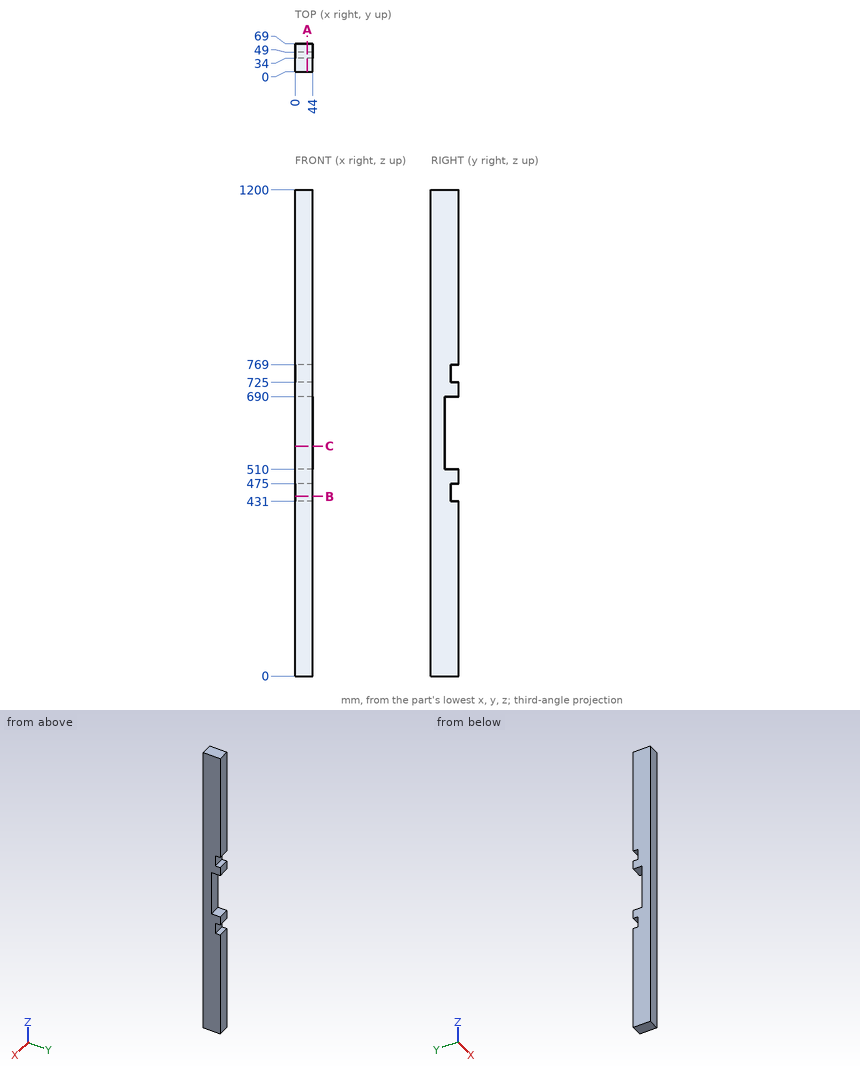
For this review, use the dimensioned drawing (mm, ordinates from the lowest corner) and the shaded views. Coordinates: 2 decimals unless noted, no trailing zeros. Write each loop counter-clockwise with the first axis right and the second up, starting at its lowest first coordinate (ties: lowest second). Pieces come first, ordered by that corner, then holes. Notation, with made-up numbers: (87, 4) -> (94, 4) arc R35 cw to (94, 43) -> close; hole circle Ø1 at (76.5, 12.25). An arc over 180 degrees is marked (long way). Write each question's results on one line, items separated by ' | '. Start each with the question number.
(1) Take a section at A-A on x = 30.5. Write out the cut boundary in (y, z), and give its area (3 significant figures).
(2) Take a section at B-B on z = 443.5. Write out the cut boundary in (x, y), and give its area (3 significant figures).
(3) For line 1 along Z through (x, y) = (34, 56); line 2 along Z through (x, y) = (2.5, 44.5); line 3 along Y through (x, z) = (11.5, 467), list the stretches that pass through material, from the lowest coordinate up. Write a range as from..to.
(4) Take a section at C-C on z = 567.5. Write out the cut boundary in (x, y), and give its area (3 significant figures).
(5) Clearance check with flat-ended pins moving along their axes: P1, Ø13, axis at x = 23.5, z = 558.5, coming from the +Y side; P2, Ø13, axis at x = 23, z = 444, coming from the +Y side. State where each tip first meets the part, or that it passes through.
Results found:
1) outline: (0, 0) -> (69, 0) -> (69, 431) -> (49, 431) -> (49, 475) -> (69, 475) -> (69, 510) -> (34, 510) -> (34, 690) -> (69, 690) -> (69, 725) -> (49, 725) -> (49, 769) -> (69, 769) -> (69, 1200) -> (0, 1200) -> close | area: 74,700 mm2
2) outline: (0, 0) -> (44, 0) -> (44, 49) -> (0, 49) -> close | area: 2,160 mm2
3) line 1: z = 0..431, 475..510, 690..725, 769..1200 | line 2: z = 0..510, 690..1200 | line 3: y = 0..49
4) outline: (0, 0) -> (44, 0) -> (44, 34) -> (0, 34) -> close | area: 1,500 mm2
5) P1: stops at y = 34 | P2: stops at y = 49
